Autodesk Inventor part; units mm, degrees
ref_plane "YZ Plane" through (0, 0, 0) normal (1, 0, 0) x (0, 1, 0)
ref_plane "XZ Plane" through (0, 0, 0) normal (0, 1, 0) x (-1, 0, 0)
ref_plane "XY Plane" through (0, 0, 0) normal (0, 0, 1) x (1, 0, 0)
sketch "Sketch2" plane through (0, 0, 0) normal (1, 0, 0) x (0, 1, 0)
  line L0 (13.4931, 0) -> (24.25, 0)
  line L1 (24.25, 0) -> (24.25, -1)
  line L2 (24.25, -1) -> (23.7248, -1.75)
  line L3 (23.7248, -1.75) -> (23.7248, -2)
  line L4 (23.7248, -2) -> (23, -2)
  line L5 (0, 0) -> (0, -8.2884)
  line L6 (23, -2) -> (23, -1)
  line L7 (23, -1) -> (3.7625, -1)
  line L8 (13.4931, 0) -> (3.7625, 0)
  line L9 (3.7625, 0) -> (3.7625, -1)
  dimension "d3" = 1
  dimension "d4" = 145
  dimension "d5" = 0.75
  dimension "d7" = 0.25
  dimension "d8" = 2
  dimension "d10" = 48.5
  dimension "d11" = 47.4497
  dimension "d12" = 1.25
  dimension "d13" = 7.525
revolve "Revolution1" add sketch "Sketch2" angle 360 about axis through (0, 0, 0) along (0, 0, -1)
sketch "Sketch3" plane through (0, 0, 0) normal (0, 0, 1) x (1, 0, 0)
  circle A0 centre (0, 0) radius 3.7625
  circle A1 centre (0, 0) radius 3.7625
  circle A2 centre (0, 0) radius 24.25
  point P0 (0, 0)
  point P1 (0, 0)
  point P2 (0, 19.5)
  dimension "d15" = 19.5
  dimension "d16" = 48.5
hole "Hole1" at (0, 0, 0) at (0, 19.5, 0) direction (0, 0, -1) diameter 5 end through all
pattern_circular "Circular Pattern1" count 6 over 360 about axis through (0, 0, -10) along (0, 0, 1) of "Hole1"
chamfer "Chamfer1" distance 0.25 angle 45 2 edges at (0, -3.7625, 0) (0, -3.7625, -1)
properties part number "Front cover of servo motor" material "Aluminum 6061-AHC"
CAD build for the part. Positions are in the model's coordinates, mm. A direction names the side the tool comes from. Round coordinates to 2 decimals unless told otherwise and drop trailing zeros. Order: outer loops, then holes, each group sorted by start corner. A loop starts at its lowest first (then second) coordinate and runs counter-clockwise, first axis right, second up.
Item 1: Probe line 1 along X through (y, z) = (0, -0.45); line 2 along X through (y, z) = (9.75, -0.45); line 3 along Z through (x, y) = (11, 16.5). List the from-to ranges inside material, lowest first.
Item 2: Saw through at C-C on y = -9.75. State how many separate pieces and enclosed holes the cut face has, then the cut area to 3 significant figures.
Item 3: Pin check, flat tips, straight feed: pin 1 (4 mm diameter, centred on x = 0, y = -19.5, fed in from +Z); pin 2 (5 mm diameter, centred on x = -5.5, y = -16.5, fed in from -Z). Stop position of each tip, or through.
Item 4: Saw through at D-D on z = -1.35. Write the cut outline in (x, y).
Item 5: Tool access for faces 1 (the face through (-22.804, -2.994, -1.493)), 2 (the face through (17.638, 12.135, -0.507)): list every direction of +Z, -Z, +X, -X, +Y, -Y with a clear straight run to the whole face (end or side of a thin tool).
Item 6: Saw through at B-B on x = 0. Write the cut outline in (y, z).
Item 7: Saw through at A-A on y = 0. Write the cut outline in (x, z), then the cut area to 3 significant figures.
Item 8: Mould opens along X. For faces 3 (the face through (19.105, -10.904, -0.507)), 4 (the face through (-5, 0, 0)), 5 (the face through (-21.514, 11.19, -0.507)) say: pulls with the +X half, pulls with the -X half, needs draft (parallel to the pull), parting line crosses it, or undercut.
Reported:
1. line 1: x = -24.25 to -3.76, 3.76 to 24.25
1. line 2: x = -22.2 to -19.39, -14.39 to 14.39, 19.39 to 22.2
1. line 3: z = -1 to 0
2. separate pieces: 3
2. enclosed holes: 0
2. area: 36.4 mm2
3. pin 1: passes through
3. pin 2: stops at z = -1
4. outline: circle Ø48.01 at (0, 0); hole circle Ø46 at (0, 0)
5. face 1: -Z
5. face 2: +Z, -Z
6. outline: (-24.25, -1) - (-23.72, -1.75) - (-23.72, -2) - (-23, -2) - (-23, -1) - (-22, -1) - (-22, 0) - (-24.25, 0) - close; (-17, -1) - (-4.01, -1) - (-3.76, -0.75) - (-3.76, -0.25) - (-4.01, 0) - (-17, 0) - close; (3.76, -0.75) - (4.01, -1) - (17, -1) - (17, 0) - (4.01, 0) - (3.76, -0.25) - close; (22, -1) - (23, -1) - (23, -2) - (23.72, -2) - (23.72, -1.75) - (24.25, -1) - (24.25, 0) - (22, 0) - close
7. outline: (-24.25, -1) - (-23.72, -1.75) - (-23.72, -2) - (-23, -2) - (-23, -1) - (-4.01, -1) - (-3.76, -0.75) - (-3.76, -0.25) - (-4.01, 0) - (-24.25, 0) - close; (3.76, -0.75) - (4.01, -1) - (23, -1) - (23, -2) - (23.72, -2) - (23.72, -1.75) - (24.25, -1) - (24.25, 0) - (4.01, 0) - (3.76, -0.25) - close
7. area: 42.7 mm2
8. face 3: undercut
8. face 4: needs draft
8. face 5: parting line crosses it
